CAD build for the part. Positions are in the model's coordinates, mm. Face numbers are marked on the shaded views. A direction names the side the tool comes from. Round coordinates to 2 decimals unless told otherwise and drop trailing zeros. Write each loop counter-clockwise with the first axis right and the second up, starting at its lowest first coordinate (ties: lowest second). Pieces come first, ordered by that corner, then holes. Notation, with made-up numbers: (80, -14) - (105, -14) arc R22 ccw to (105, 22) - close; hole circle Ø3 at (62, 58.5). An arc over 180 degrees is marked (long way). Answer in a Markdown table with one row per item.
```python
from build123d import *

# Parameters (mm, degrees)
F0_W     = 21.6265451163
F0_H     = 44.9824891984
F0_R     = 0.5
F0_R_2   = 1.7272
F0_R_3   = 2.085
F1_DEPTH = 15
F2_DEPTH = 3.2


# Not quite as in the source:
# - a feature names something its author has since deleted; it is built from what else it names


with BuildPart() as f1:
    # F0 (on Top) → F1 (new body)
    with BuildSketch(Plane.XY):
        Rectangle(F0_W, F0_H)
        Polygon((-4.9074772881, -12.4994842336), (-2.4537386441, -8.2494842336), (2.4537386441, -8.2494842336), (4.9074772881, -12.4994842336), (2.4537386441, -16.7494842336), (-2.4537386441, -16.7494842336), align=None, mode=Mode.SUBTRACT)
        Circle(F0_R, mode=Mode.SUBTRACT)
        with Locations((0, 12.0378434658)):
            Circle(F0_R_2, mode=Mode.SUBTRACT)
        Polygon((2.4537386441, -8.2494842336), (-2.4537386441, -8.2494842336), (-4.9074772881, -12.4994842336), (-2.4537386441, -16.7494842336), (2.4537386441, -16.7494842336), (4.9074772881, -12.4994842336), align=None)
        with Locations((0, -12.4994842336)):
            Circle(F0_R_3, mode=Mode.SUBTRACT)
    extrude(amount=-F1_DEPTH)

    # F0 (on Top) → F2 (cut)
    with BuildSketch(Plane.XY):
        Polygon((2.4537386441, -8.2494842336), (-2.4537386441, -8.2494842336), (-4.9074772881, -12.4994842336), (-2.4537386441, -16.7494842336), (2.4537386441, -16.7494842336), (4.9074772881, -12.4994842336), align=None)
        with Locations((0, -12.4994842336)):
            Circle(F0_R_3, mode=Mode.SUBTRACT)
    extrude(amount=-F2_DEPTH, mode=Mode.SUBTRACT)


solid = f1.part
```
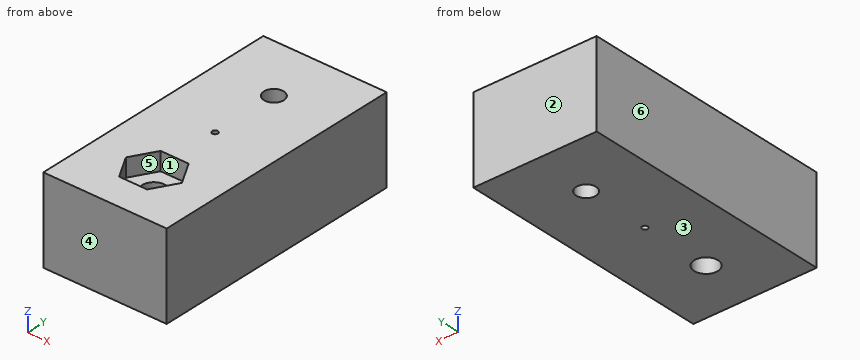
Q1. Drill centre lines: line 1 (Y direction, x = 0, z = -5); line 2 (Y direction, x = -4.25, z = -2.75); line 3 (X direction, y = -13.5, z = -9). Where is each one in solid material? Low to high.
Computed:
| item | result |
|---|---|
| line 1 | y = -22.49 to -14.58, -10.41 to -0.5, 0.5 to 10.31, 13.77 to 22.49 |
| line 2 | y = -22.49 to -13.64, -11.36 to 22.49 |
| line 3 | x = -10.81 to -1.83, 1.83 to 10.81 |
Q2. Saw through at A-A on y = 0. List the corners of the cut face in (x, z).
Computed:
| item | result |
|---|---|
| outline | (-10.81, -15) - (-0.5, -15) - (-0.5, 0) - (-10.81, 0) - close; (0.5, -15) - (10.81, -15) - (10.81, 0) - (0.5, 0) - close |
Q3. Saw through at B-B on x = 0. List the corners of the cut face in (y, z).
Computed:
| item | result |
|---|---|
| outline | (-22.49, -15) - (-14.58, -15) - (-14.58, -3.2) - (-16.75, -3.2) - (-16.75, 0) - (-22.49, 0) - close; (-10.41, -15) - (-0.5, -15) - (-0.5, 0) - (-8.25, 0) - (-8.25, -3.2) - (-10.41, -3.2) - close; (0.5, -15) - (10.31, -15) - (10.31, 0) - (0.5, 0) - close; (13.77, -15) - (22.49, -15) - (22.49, 0) - (13.77, 0) - close |
Q4. Saw through at C-C on z = -1.25. List the corners of the cut face in (x, y).
Computed:
| item | result |
|---|---|
| outline | (-10.81, -22.49) - (10.81, -22.49) - (10.81, 22.49) - (-10.81, 22.49) - close; hole (-4.91, -12.5) - (-2.45, -16.75) - (2.45, -16.75) - (4.91, -12.5) - (2.45, -8.25) - (-2.45, -8.25) - close; hole circle Ø3.45 at (0, 12.04); hole circle Ø1 at (0, 0) |
Q5. Flat gauge pin, fed straight in: pin 1 (2.5 mm diameter, centred on x = 0, y = -12.5, fed in from +Z). Where does the tip first touch, or does it go through?
Computed:
| item | result |
|---|---|
| pin 1 | passes through |
Q6. Saw through at D-D on x = -3.5. List the corners of the cut face in (y, z), then the cut area to 3 significant figures.
Computed:
| item | result |
|---|---|
| outline | (-22.49, -15) - (22.49, -15) - (22.49, 0) - (-10.06, 0) - (-10.06, -3.2) - (-14.94, -3.2) - (-14.94, 0) - (-22.49, 0) - close |
| area | 659 mm2 |
Q7. Pull direction Y, two halves, no side cores. Call the marked faces 1, 2, 3 and 4: released by +Y, released by -Y, zero draft, split by the parting line, or undercut.
Computed:
| item | result |
|---|---|
| face 1 | undercut |
| face 2 | released by +Y |
| face 3 | zero draft |
| face 4 | released by -Y |
Q8. 3-axis set-ups, long thin cutter, end or side, ignore diameter. For the marked faces 5 and 6: which of +Z, -Z, +X, -X, +Y, -Y reach the whole face in a straight line?
Computed:
| item | result |
|---|---|
| face 5 | +Z |
| face 6 | +Z, -Z, -X, +Y, -Y |
